Geometry check sheet. Reference: the model listing, model coordinates, mm. A direction names the side the tool comes from. Give positions to 0.01 mm unless a question says otherwise; leave off trailing zeros. Loops run counter-clockwise (first coordinate to the right, second up) from the corner with the lowest first, then second, coordinate; pieces in that order, holes last. Notation, with made-up numbers: (47.25, 2) -> (88.25, 2) arc R12 ccw to (88.25, 25) -> close; hole circle Ø10 at (6, 58). An arc over 180 degrees is marked (long way). Write item = value, one per line.
```python
from build123d import *

# Parameters (mm, degrees)
F1_DEPTH    = 101.6
F2_T1_DEPTH = 101.6
F2_T3_DEPTH = 213.9945264783
F3_R        = 1.651
F4_DEPTH    = 127
F5_R        = 3.81
F5_R_2      = 1.651
F6_DEPTH    = 98.425


# Not quite as in the source:
# - a fillet or chamfer that OpenCascade refuses, or shapes differently, is made with other operations: its cross-section is extruded or revolved along the edge and cut away or added


with BuildPart() as f1:
    # F0 (on Front) → F1 (new body)
    with BuildSketch(Plane.XZ):
        with BuildLine():
            ThreePointArc((36.7729649274, -9.9679010051), (37.7667841081, -5.0279238392), (38.1, 0))
            ThreePointArc((38.1, 0), (37.363123518, 7.4570101903), (35.1809973239, 14.6255744261))
            ThreePointArc((35.1809973239, 14.6255744261), (34.1844683928, 16.823558503), (33.0507832594, 18.9540424696))
            ThreePointArc((33.0507832594, 18.9540424696), (25.1442335653, 28.6247710631), (14.5348789212, 35.2185646321))
            ThreePointArc((14.5348789212, 35.2185646321), (12.2760171106, 36.068121713), (9.9679010051, 36.7729649274))
            ThreePointArc((9.9679010051, 36.7729649274), (-2.4611116668, 38.0204277904), (-14.6255744261, 35.1809973239))
            ThreePointArc((-14.6255744261, 35.1809973239), (-16.823558503, 34.1844683928), (-18.9540424696, 33.0507832594))
            ThreePointArc((-18.9540424696, 33.0507832594), (-28.6247710631, 25.1442335653), (-35.2185646321, 14.5348789212))
            ThreePointArc((-35.2185646321, 14.5348789212), (-36.068121713, 12.2760171106), (-36.7729649274, 9.9679010051))
            ThreePointArc((-36.7729649274, 9.9679010051), (-38.0204277904, -2.4611116668), (-35.1809973239, -14.6255744261))
            ThreePointArc((-35.1809973239, -14.6255744261), (-34.1844683928, -16.823558503), (-33.0507832594, -18.9540424696))
            ThreePointArc((-33.0507832594, -18.9540424696), (-25.1442335653, -28.6247710631), (-14.5348789212, -35.2185646321))
            ThreePointArc((-14.5348789212, -35.2185646321), (-12.2760171106, -36.068121713), (-9.9679010051, -36.7729649274))
            ThreePointArc((-9.9679010051, -36.7729649274), (2.4611116668, -38.0204277904), (14.6255744261, -35.1809973239))
            ThreePointArc((14.6255744261, -35.1809973239), (16.823558503, -34.1844683928), (18.9540424696, -33.0507832594))
            ThreePointArc((18.9540424696, -33.0507832594), (28.6247710631, -25.1442335653), (35.2185646321, -14.5348789212))
            ThreePointArc((35.2185646321, -14.5348789212), (36.068121713, -12.2760171106), (36.7729649274, -9.9679010051))
        make_face()
        with BuildLine():
            ThreePointArc((-35.2185646321, 14.5348789212), (-28.6247710631, 25.1442335653), (-18.9540424696, 33.0507832594))
            Line((-18.9540424696, 33.0507832594), (-23.9079516621, 45.688308647))
            Line((-23.9079516621, 45.688308647), (-66.712088778, 28.9090894698))
            Line((-66.712088778, 28.9090894698), (-41.705504873, 27.890755436))
            Line((-41.705504873, 27.890755436), (-35.2185646321, 14.5348789212))
        make_face()
        with BuildLine():
            ThreePointArc((-14.6255744261, 35.1809973239), (-2.4611116668, 38.0204277904), (9.9679010051, 36.7729649274))
            Line((9.9679010051, 36.7729649274), (15.4010381207, 49.2119876098))
            Line((15.4010381207, 49.2119876098), (-26.7307571601, 67.6143835641))
            Line((-26.7307571601, 67.6143835641), (-9.7685030073, 49.2119876098))
            Line((-9.7685030073, 49.2119876098), (-14.6255744261, 35.1809973239))
        make_face()
        with BuildLine():
            ThreePointArc((14.5348789212, 35.2185646321), (25.1442335653, 28.6247710631), (33.0507832594, 18.9540424696))
            Line((33.0507832594, 18.9540424696), (45.688308647, 23.9079516621))
            Line((45.688308647, 23.9079516621), (28.9090894698, 66.712088778))
            Line((28.9090894698, 66.712088778), (27.890755436, 41.705504873))
            Line((27.890755436, 41.705504873), (14.5348789212, 35.2185646321))
        make_face()
        with BuildLine():
            ThreePointArc((35.1809973239, 14.6255744261), (37.363123518, 7.4570101903), (38.1, 0))
            ThreePointArc((38.1, 0), (37.7667841081, -5.0279238392), (36.7729649274, -9.9679010051))
            Line((36.7729649274, -9.9679010051), (49.2119876098, -15.4010381207))
            Line((49.2119876098, -15.4010381207), (67.6143835641, 26.7307571601))
            Line((67.6143835641, 26.7307571601), (49.2119876098, 9.7685030073))
            Line((49.2119876098, 9.7685030073), (35.1809973239, 14.6255744261))
        make_face()
        with BuildLine():
            Line((41.705504873, -27.890755436), (35.2185646321, -14.5348789212))
            ThreePointArc((35.2185646321, -14.5348789212), (28.6247710631, -25.1442335653), (18.9540424696, -33.0507832594))
            Line((18.9540424696, -33.0507832594), (23.9079516621, -45.688308647))
            Line((23.9079516621, -45.688308647), (66.712088778, -28.9090894698))
            Line((66.712088778, -28.9090894698), (41.705504873, -27.890755436))
        make_face()
        with BuildLine():
            Line((9.7685030073, -49.2119876098), (14.6255744261, -35.1809973239))
            ThreePointArc((14.6255744261, -35.1809973239), (2.4611116668, -38.0204277904), (-9.9679010051, -36.7729649274))
            Line((-9.9679010051, -36.7729649274), (-15.4010381207, -49.2119876098))
            Line((-15.4010381207, -49.2119876098), (26.7307571601, -67.6143835641))
            Line((26.7307571601, -67.6143835641), (9.7685030073, -49.2119876098))
        make_face()
        with BuildLine():
            Line((-27.890755436, -41.705504873), (-14.5348789212, -35.2185646321))
            ThreePointArc((-14.5348789212, -35.2185646321), (-25.1442335653, -28.6247710631), (-33.0507832594, -18.9540424696))
            Line((-33.0507832594, -18.9540424696), (-45.688308647, -23.9079516621))
            Line((-45.688308647, -23.9079516621), (-28.9090894698, -66.712088778))
            Line((-28.9090894698, -66.712088778), (-27.890755436, -41.705504873))
        make_face()
        with BuildLine():
            ThreePointArc((-35.1809973239, -14.6255744261), (-38.0204277904, -2.4611116668), (-36.7729649274, 9.9679010051))
            Line((-36.7729649274, 9.9679010051), (-49.2119876098, 15.4010381207))
            Line((-49.2119876098, 15.4010381207), (-67.6143835641, -26.7307571601))
            Line((-67.6143835641, -26.7307571601), (-49.2119876098, -9.7685030073))
            Line((-49.2119876098, -9.7685030073), (-35.1809973239, -14.6255744261))
        make_face()
    extrude(amount=F1_DEPTH)

    # F2: fillet of radius 25.4 on 16 edges, made by hand

    # F2_s2 → F2_t1 (join)
    with BuildSketch(Plane.XZ):
        with BuildLine():
            ThreePointArc((-56.8805102577, 28.5087216686), (-44.1451035636, 24.4740120759), (-35.2185646321, 14.5348789212))
            Line((-35.2185646321, 14.5348789212), (-41.705504873, 27.890755436))
            Line((-41.705504873, 27.890755436), (-56.8805102577, 28.5087216686))
        make_face()
        with BuildLine():
            ThreePointArc((-60.3793049354, -20.0618841058), (-48.5210419877, -13.9095621843), (-35.1809973239, -14.6255744261))
            Line((-35.1809973239, -14.6255744261), (-49.2119876098, -9.7685030073))
            Line((-49.2119876098, -9.7685030073), (-60.3793049354, -20.0618841058))
        make_face()
        with BuildLine():
            ThreePointArc((-28.5087216686, -56.8805102577), (-24.4740120759, -44.1451035636), (-14.5348789212, -35.2185646321))
            Line((-14.5348789212, -35.2185646321), (-27.890755436, -41.705504873))
            Line((-27.890755436, -41.705504873), (-28.5087216686, -56.8805102577))
        make_face()
        with BuildLine():
            ThreePointArc((20.0618841058, -60.3793049354), (13.9095621843, -48.5210419877), (14.6255744261, -35.1809973239))
            Line((14.6255744261, -35.1809973239), (9.7685030073, -49.2119876098))
            Line((9.7685030073, -49.2119876098), (20.0618841058, -60.3793049354))
        make_face()
        with BuildLine():
            ThreePointArc((56.8805102577, -28.5087216686), (44.1451035636, -24.4740120759), (35.2185646321, -14.5348789212))
            Line((35.2185646321, -14.5348789212), (41.705504873, -27.890755436))
            Line((41.705504873, -27.890755436), (56.8805102577, -28.5087216686))
        make_face()
        with BuildLine():
            ThreePointArc((60.3793049354, 20.0618841058), (48.5210419877, 13.9095621843), (35.1809973239, 14.6255744261))
            Line((35.1809973239, 14.6255744261), (49.2119876098, 9.7685030073))
            Line((49.2119876098, 9.7685030073), (60.3793049354, 20.0618841058))
        make_face()
        with BuildLine():
            ThreePointArc((28.5087216686, 56.8805102577), (24.4740120759, 44.1451035636), (14.5348789212, 35.2185646321))
            Line((14.5348789212, 35.2185646321), (27.890755436, 41.705504873))
            Line((27.890755436, 41.705504873), (28.5087216686, 56.8805102577))
        make_face()
        with BuildLine():
            ThreePointArc((-20.0618841058, 60.3793049354), (-13.9095621843, 48.5210419877), (-14.6255744261, 35.1809973239))
            Line((-14.6255744261, 35.1809973239), (-9.7685030073, 49.2119876098))
            Line((-9.7685030073, 49.2119876098), (-20.0618841058, 60.3793049354))
        make_face()
    extrude(amount=F2_T1_DEPTH)

    # F2_s4 → F2_t3 (cut)
    with BuildSketch(Plane.XZ.offset(-56.1972632391)):
        with BuildLine():
            ThreePointArc((-36.7729649274, 9.9679010051), (-49.6032208566, 5.3697394136), (-58.2095345387, -5.1986058702))
            Line((-58.2095345387, -5.1986058702), (-49.2119876098, 15.4010381207))
            Line((-49.2119876098, 15.4010381207), (-36.7729649274, 9.9679010051))
        make_face()
        with BuildLine():
            ThreePointArc((-18.9540424696, 33.0507832594), (-31.2777946839, 38.8717529889), (-44.8363260656, 37.4843871385))
            Line((-44.8363260656, 37.4843871385), (-23.9079516621, 45.688308647))
            Line((-23.9079516621, 45.688308647), (-18.9540424696, 33.0507832594))
        make_face()
        with BuildLine():
            ThreePointArc((9.9679010051, 36.7729649274), (5.3697394136, 49.6032208566), (-5.1986058702, 58.2095345387))
            Line((-5.1986058702, 58.2095345387), (15.4010381207, 49.2119876098))
            Line((15.4010381207, 49.2119876098), (9.9679010051, 36.7729649274))
        make_face()
        with BuildLine():
            ThreePointArc((33.0507832594, 18.9540424696), (38.8717529889, 31.2777946839), (37.4843871385, 44.8363260656))
            Line((37.4843871385, 44.8363260656), (45.688308647, 23.9079516621))
            Line((45.688308647, 23.9079516621), (33.0507832594, 18.9540424696))
        make_face()
        with BuildLine():
            ThreePointArc((36.7729649274, -9.9679010051), (49.6032208566, -5.3697394136), (58.2095345387, 5.1986058702))
            Line((58.2095345387, 5.1986058702), (49.2119876098, -15.4010381207))
            Line((49.2119876098, -15.4010381207), (36.7729649274, -9.9679010051))
        make_face()
        with BuildLine():
            ThreePointArc((18.9540424696, -33.0507832594), (31.2777946839, -38.8717529889), (44.8363260656, -37.4843871385))
            Line((44.8363260656, -37.4843871385), (23.9079516621, -45.688308647))
            Line((23.9079516621, -45.688308647), (18.9540424696, -33.0507832594))
        make_face()
        with BuildLine():
            ThreePointArc((-9.9679010051, -36.7729649274), (-5.3697394136, -49.6032208566), (5.1986058702, -58.2095345387))
            Line((5.1986058702, -58.2095345387), (-15.4010381207, -49.2119876098))
            Line((-15.4010381207, -49.2119876098), (-9.9679010051, -36.7729649274))
        make_face()
        with BuildLine():
            ThreePointArc((-33.0507832594, -18.9540424696), (-38.8717529889, -31.2777946839), (-37.4843871385, -44.8363260656))
            Line((-37.4843871385, -44.8363260656), (-45.688308647, -23.9079516621))
            Line((-45.688308647, -23.9079516621), (-33.0507832594, -18.9540424696))
        make_face()
    extrude(amount=F2_T3_DEPTH, mode=Mode.SUBTRACT)

    # F3 (on face) → F4 (cut)
    with BuildSketch(Plane(origin=(0, 0, 0), x_dir=(-1, 0, 0), z_dir=(0, 1, 0))):
        with Locations((0, 10.5664)):
            Circle(F3_R)
        with Locations((-10.5664, 0)):
            Circle(F3_R)
        with Locations((10.5664, 0)):
            Circle(F3_R)
        with Locations((0, -10.5664)):
            Circle(F3_R)
    extrude(amount=-F4_DEPTH, mode=Mode.SUBTRACT)

    # F5 (on face) → F6 (cut)
    with BuildSketch(Plane(origin=(0, 0, 0), x_dir=(-1, 0, 0), z_dir=(0, 1, 0))):
        with Locations((0, 10.5664)):
            Circle(F5_R)
        with Locations((0, 10.5664)):
            Circle(F5_R_2, mode=Mode.SUBTRACT)
        with Locations((10.5664, 0)):
            Circle(F5_R)
        with Locations((10.5664, 0)):
            Circle(F5_R_2, mode=Mode.SUBTRACT)
        with Locations((0, -10.5664)):
            Circle(F5_R)
        with Locations((0, -10.5664)):
            Circle(F5_R_2, mode=Mode.SUBTRACT)
        with Locations((-10.5664, 0)):
            Circle(F5_R)
        with Locations((-10.5664, 0)):
            Circle(F5_R_2, mode=Mode.SUBTRACT)
    extrude(amount=-F6_DEPTH, mode=Mode.SUBTRACT)


solid = f1.part
```
Item 1: Thickness scan on L1, parallel to Z at x = 0, y = -56.5; L2, parallel to Z at x = 0, y = -99.7; L3, parallel to Z at x = -47.5, y = -55. Record the ranges inside material, lowest first. Write a range as [from, to].
Answer:
L1 = [-55.16, -14.38], [-6.76, 6.76], [14.38, 55.16]
L2 = [-55.16, -12.22], [-8.92, 8.92], [12.22, 55.16]
L3 = [-13.71, 6.71], [26.3, 36.44]
Item 2: Gauge pin test, flat ends, axial feed: pin 1 (9 mm diameter, centred on x = 10.57, z = 0, fed in from -Y); pin 2 (2.5 mm diameter, centred on x = -10.5, z = -1.5, fed in from +Y) (3 decimals); pin 3 (1.5 mm diameter, centred on x = 41, y = -74, fed in from +Z); pin 4 (1 mm diameter, centred on y = -89, z = 40.5, fed in from +X). Record the tip position at first contact, or that the pin passes through.
Answer:
pin_1 = -101.6
pin_2 = -98.425
pin_3 = 13.51
pin_4 = 38.85
Item 3: Tool access check on faces 4 (the flat face through (-61.87, -50.09, 28.71)), 5 (the flat face through (-64, -50.1, -23.4)), 6 (the flat face through (55.621, -50.089, -33.257)), 7 (the flat face through (9, -98.425, -1)), 8 (the cylindrical face through (16.79, -50.09, -34.2)). Record the directions out of +Z, -Z, +X, -X, +Y, -Y that give a thin tool (end or side, any length) a straight path to the whole face; none if there is none.
Answer:
face_4 = -X, +Y, -Y
face_5 = -Z, +Y, -Y
face_6 = -Z, +X, +Y, -Y
face_7 = +Y
face_8 = +Y, -Y
Item 4: Section check A-A, the plane x = -42. Record the cut outline in (y, z), plus the area to 3 significant figures.
Answer:
outline = (-101.6, -13.37) -> (0, -13.37) -> (0, 9.03) -> (-101.6, 9.03) -> close; (-101.6, 22.93) -> (0, 22.93) -> (0, 38.41) -> (-101.6, 38.41) -> close
area = 3,850 mm^2
Item 5: Section check C-C, the plane y = -80.5. Give the number of separate pieces and of enclosed holes in the cut face, plus the area to 3 significant figures.
Answer:
separate_pieces = 1
enclosed_holes = 4
area = 8,170 mm^2
Item 6: Section check B-B, the plane z = -53. Record the cut outline in (x, y).
Answer:
outline = (-34.28, -101.6) -> (-28.05, -101.6) -> (-28.05, 0) -> (-34.28, 0) -> close; (-2.49, -101.6) -> (15.32, -101.6) -> (15.32, 0) -> (-2.49, 0) -> close
Item 7: Draft check along X on faces 1 (the flat face through (-1, 0, 1)), 2 (the cylindrical face through (-34.2, -50.09, -16.79)), 3 (the flat face through (62.846, -50.089, 15.814)). Enter one of: +X half, -X half, draft (parallel to the pull), parting line (faces both ways), or undercut.
Answer:
face_1 = draft
face_2 = undercut
face_3 = +X half
